For this review, take the finished solid that the model builds, in its own axes (mm). Face numbers are marked on the shaded views. A direction names the side the tool comes from. Coordinates: 2 decimals unless noted, no trailing zeros. Loops run counter-clockwise (first coordinate to the right, second up) from the corner with the lowest first, then second, coordinate; pieces in that order, holes last. Notation, with made-up numbers: (82.25, -0.75) - (88.25, -0.75) arc R17 cw to (88.25, 4.25) - close; hole circle Ø4 at (-21, 39.25). An arc over 180 degrees is marked (long way). One line per item, written item: value. Start each with the question number.
1. Take a section at B-B, the plane y = 21.5. State the section outline as (x, z) points.
2. Insertion check: pin 1 (2 mm diameter, centred on x = 34.5, z = 29, fed in from +Y); pin 2 (1.5 mm diameter, centred on x = -58, z = 51.5, fed in from -Y); pin 3 (3 mm diameter, centred on x = 0, y = 70.16, fed in from -Z); pin 4 (12 mm diameter, centred on y = 4.5, z = 76.5, fed in from -X). Each pin has a flat end and moves straight along its axis. Give the tip position at first contact, or say it passes through.
3. Take a section at C-C, the plane z = 50. State the section outline as (x, y) points, and give its area (3 significant figures).
4. Take a section at D-D, the plane y = -70. State the section outline as (x, z) points.
5. The part is to be moulded in two halves that separate along X. For the marked faces 1, 2 and 3, say which applies: released by +X, released by -X, zero draft, split by the parting line, or undercut.
6. To check wall thickness, follow line 1 (Y direction, x = 0, z = 8); line 2 (Z direction, x = 13, y = -53); line 3 (Y direction, x = -4.5, z = 64). State the ranges of each line that lie inside material, in increasing order. Write a range as from..to.
7. For the marked faces 4 and 5, list the 3-axis set-ups (+Z, -Z, +X, -X, +Y, -Y) from which the entire face can be reached by the end or side of a thin tool; tool diameter is ignored.
8. Take a section at A-A, the plane x = 0. State the section outline as (y, z) points, and give its area (3 significant figures).
```python
from build123d import *

# Parameters (mm, degrees)
SKETCH2_R           = 75
BOSS_EXTRUDE1_DEPTH = 85
SKETCH4_R           = 65
CUT_EXTRUDE2_DEPTH  = 25
SKETCH5_R           = 55
CUT_EXTRUDE3_DEPTH  = 50
SKETCH7_R           = 2.5
CUT_EXTRUDE4_DEPTH  = 20
CIRPATTERN1_COUNT   = 5
SKETCH8_R           = 2.5
CUT_EXTRUDE5_DEPTH  = 10
CIRPATTERN2_COUNT   = 4


with BuildPart() as part:
    # Sketch2 → Boss-Extrude1 (new body)
    with BuildSketch(Plane(origin=(0, 0, 0), x_dir=(0, 1, 0), z_dir=(0, 0, 1))):
        with Locations(Location((0, 0, 0), (0, 0, 270))):
            Circle(SKETCH2_R)
    extrude(amount=BOSS_EXTRUDE1_DEPTH)

    # Sketch4 → Cut-Extrude2 (cut)
    with BuildSketch(Plane.XY.offset(85)):
        Circle(SKETCH4_R)
    extrude(amount=-CUT_EXTRUDE2_DEPTH, mode=Mode.SUBTRACT)

    # Sketch5 → Cut-Extrude3 (cut)
    with BuildSketch(Plane.XY.offset(60)):
        Circle(SKETCH5_R)
    extrude(amount=-CUT_EXTRUDE3_DEPTH, mode=Mode.SUBTRACT)

    # Sketch7 → Cut-Extrude4 (cut)
    with BuildSketch(Plane.XY.offset(85)):
        with Locations((0, 69.72339814)):
            Circle(SKETCH7_R)
    cut_extrude4 = extrude(amount=-CUT_EXTRUDE4_DEPTH, mode=Mode.SUBTRACT)

    # CirPattern1: Cut-Extrude4 ×5 about axis
    cirpattern1_axis = Axis((0, 0, 0), (0, 0, 1))
    for i in range(1, CIRPATTERN1_COUNT):
        add(cut_extrude4.rotate(cirpattern1_axis, i * 360 / CIRPATTERN1_COUNT), mode=Mode.SUBTRACT)

    # Sketch8 → Cut-Extrude5 (cut)
    with BuildSketch(Plane(origin=(0, 0, 0), x_dir=(1, 0, 0), z_dir=(0, 0, -1))):
        with Locations(Location((0, 70, 0), (0, 0, 180))):
            Circle(SKETCH8_R)
    cut_extrude5 = extrude(amount=-CUT_EXTRUDE5_DEPTH, mode=Mode.SUBTRACT)

    # CirPattern2: Cut-Extrude5 ×4 about axis
    cirpattern2_axis = Axis((0, 0.077864294, 0), (0, 0, 1))
    for i in range(1, CIRPATTERN2_COUNT):
        add(cut_extrude5.rotate(cirpattern2_axis, i * 360 / CIRPATTERN2_COUNT), mode=Mode.SUBTRACT)


solid = part.part
```
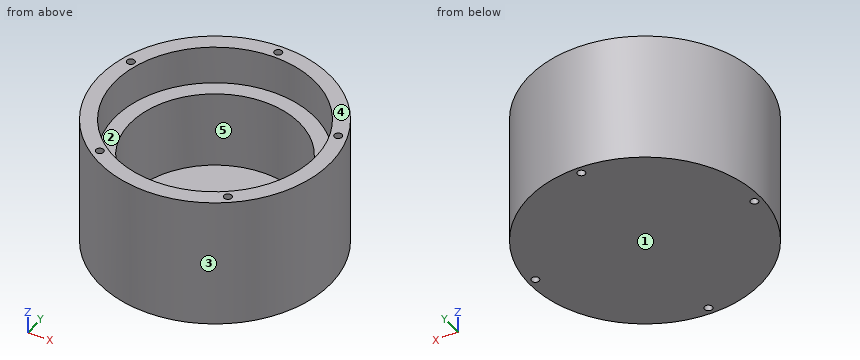
Solutions:
1. outline: (-71.85, 0) - (71.85, 0) - (71.85, 85) - (68.81, 85) - (68.81, 65) - (63.81, 65) - (63.81, 85) - (61.34, 85) - (61.34, 60) - (50.62, 60) - (50.62, 10) - (-50.62, 10) - (-50.62, 60) - (-61.34, 60) - (-61.34, 85) - (-63.81, 85) - (-63.81, 65) - (-68.81, 65) - (-68.81, 85) - (-71.85, 85) - close
2. pin 1: y = 67.1
2. pin 2: y = -48.45
2. pin 3: z = 10
2. pin 4: x = -75
3. outline: circle Ø150 at (0, 0); hole circle Ø110 at (0, 0)
3. area: 8,170 mm2
4. outline: (-26.93, 0) - (-2.5, 0) - (-2.5, 10) - (2.5, 10) - (2.5, 0) - (26.93, 0) - (26.93, 85) - (-26.93, 85) - close
5. face 1: zero draft
5. face 2: undercut
5. face 3: split by the parting line
6. line 1: -75..-72.5, -67.5..67.66, 72.66..75
6. line 2: 0..10
6. line 3: -74.86..-64.84, 64.84..74.86
7. face 4: +Z, +X, -X, +Y, -Y
7. face 5: +Z
8. outline: (-75, 0) - (-72.5, 0) - (-72.5, 10) - (-67.5, 10) - (-67.5, 0) - (67.66, 0) - (67.66, 10) - (72.66, 10) - (72.66, 0) - (75, 0) - (75, 85) - (72.22, 85) - (72.22, 65) - (67.22, 65) - (67.22, 85) - (65, 85) - (65, 60) - (55, 60) - (55, 10) - (-55, 10) - (-55, 60) - (-65, 60) - (-65, 85) - (-75, 85) - close
8. area: 3,800 mm2
